from build123d import *

# Parameters (mm, degrees)
F0_W     = 304.8
F0_H     = 50.8
F1_DEPTH = 25.4
F2_SIZE  = 6.35
F3_R     = 9.8425
F4_DEPTH = 21.59


with BuildPart() as f1:
    # F0 (on Top) → F1 (new body)
    with BuildSketch(Plane.XY):
        with Locations((-152.4, -25.4)):
            Rectangle(F0_W, F0_H)
    extrude(amount=-F1_DEPTH)

    # F2
    f2_edges = [f1.edges().sort_by_distance(p)[0] for p in [
        (0, 0, -12.7),
        (0, -50.8, -12.7),
        (-304.8, -50.8, -12.7),
        (-304.8, 0, -12.7),
    ]]
    chamfer(f2_edges, length=F2_SIZE)

    # F3 (on face) → F4 (cut)
    with BuildSketch(Plane.XY):
        with Locations((-12.7, -12.7)):
            Circle(F3_R)
        with Locations((-12.7, -38.1)):
            Circle(F3_R)
        with Locations((-38.1, -12.7)):
            Circle(F3_R)
        with Locations((-38.1, -38.1)):
            Circle(F3_R)
        with Locations((-63.5, -12.7)):
            Circle(F3_R)
        with Locations((-63.5, -38.1)):
            Circle(F3_R)
        with Locations((-88.9, -12.7)):
            Circle(F3_R)
        with Locations((-88.9, -38.1)):
            Circle(F3_R)
        with Locations((-114.3, -12.7)):
            Circle(F3_R)
        with Locations((-114.3, -38.1)):
            Circle(F3_R)
        with Locations((-139.7, -12.7)):
            Circle(F3_R)
        with Locations((-139.7, -38.1)):
            Circle(F3_R)
        with Locations((-165.1, -12.7)):
            Circle(F3_R)
        with Locations((-165.1, -38.1)):
            Circle(F3_R)
        with Locations((-190.5, -12.7)):
            Circle(F3_R)
        with Locations((-190.5, -38.1)):
            Circle(F3_R)
        with Locations((-215.9, -12.7)):
            Circle(F3_R)
        with Locations((-215.9, -38.1)):
            Circle(F3_R)
        with Locations((-241.3, -12.7)):
            Circle(F3_R)
        with Locations((-241.3, -38.1)):
            Circle(F3_R)
        with Locations((-266.7, -12.7)):
            Circle(F3_R)
        with Locations((-266.7, -38.1)):
            Circle(F3_R)
        with Locations((-292.1, -12.7)):
            Circle(F3_R)
        with Locations((-292.1, -38.1)):
            Circle(F3_R)
    extrude(amount=-F4_DEPTH, mode=Mode.SUBTRACT)


solid = f1.part
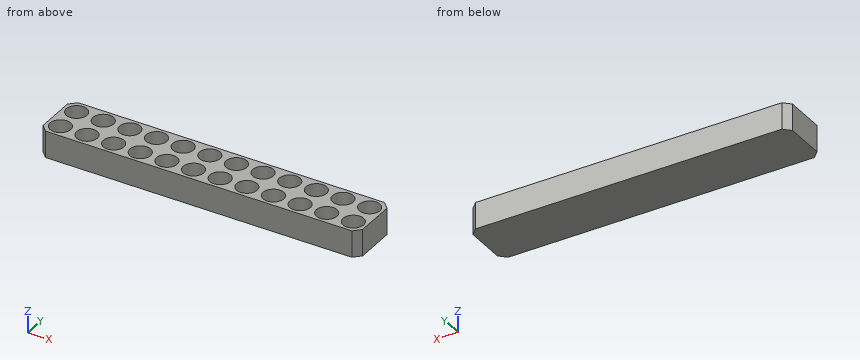
For this review, take the finished solid that the model builds, in its own axes (mm). Coordinates: 2 decimals unless noted, no trailing zeros. Loops run counter-clockwise (first coordinate to the right, second up) from the corner with the lowest first, then second, coordinate; pieces in that order, holes last. Notation, with made-up numbers: (-20, 88) - (38, 88) arc R8 cw to (38, 92) - close; hole circle Ø3 at (52, -40). An arc over 180 degrees is marked (long way). Return JSON: item names as keys, results as strings.
Item 1: For line 1 (Y direction, x = -215.9, z = -6.5); line 2 (Y direction, x = -116, z = -13.5); line 3 (Z direction, x = -122, y = -34), list the stretches that pass through material, from the lowest coordinate up.
Determined:
{"line 1": "y = -50.8 to -47.94, -28.26 to -22.54, -2.86 to 0", "line 2": "y = -50.8 to -47.79, -28.41 to -22.39, -3.01 to 0", "line 3": "z = -25.4 to -21.59"}
Item 2: Take a section at A-A (z = -8.5). State how many separate pieces and enclosed holes the cut face has, then the cut area to 3 significant figures.
Determined:
{"separate pieces": "1", "enclosed holes": "24", "area": "8,100 mm2"}
Item 3: Take a section at C-C (x = -69). Give the boundary of the cut face in (y, z).
Determined:
{"outline": "(-50.8, -25.4) - (0, -25.4) - (0, 0) - (-4.54, 0) - (-4.54, -21.59) - (-20.86, -21.59) - (-20.86, 0) - (-29.94, 0) - (-29.94, -21.59) - (-46.26, -21.59) - (-46.26, 0) - (-50.8, 0) - close"}
Item 4: Insertion check: pin 1 (10 mm diameter, centred on x = -214.5, y = -9.5, fed in from +Z). The pin has a flat end and moves straight along its axis. Give the tip position at first contact, or say it passes through.
Determined:
{"pin 1": "stops at z = -21.59"}
Item 5: Take a section at B-B (x = -139.7). Give the boundary of the cut face in (y, z).
Determined:
{"outline": "(-50.8, -25.4) - (0, -25.4) - (0, 0) - (-2.86, 0) - (-2.86, -21.59) - (-22.54, -21.59) - (-22.54, 0) - (-28.26, 0) - (-28.26, -21.59) - (-47.94, -21.59) - (-47.94, 0) - (-50.8, 0) - close"}
